Design review of the part built by this model. Coordinates are the model's own, in mm. Coordinates: 2 decimals unless noted, no trailing zeros. Write each loop counter-clockwise with the first axis right and the second up, starting at its lowest first coordinate (ties: lowest second). Pieces come first, ordered by that corner, then holes.
Q1. Add section A-A, the plane x = 0. Give the boundary of the cut face in (y, z).
Q2. To check wall thickness, follow probe 1 along Y at (x, z) = (0, 70); probe 2 along Z at (x, y) = (0, 1.25); probe 3 along Z at (x, y) = (1.5, 4). State the ranges of each line that lie inside material, in increasing order.
Q3. Add section B-B, the plane y = 5.25. Give the boundary of the cut face in (x, z).
Q4. Add section D-D, the plane z = 57. Give the boundary of the cut face in (x, y).
Q5. Clearance check with flat-ended pins moving along their axes: pin 1 Ø1.5 at (y, z) = (4, 46) entering from +X; pin 2 Ø1.5 at (y, z) = (-3, 41.5) entering from +X; pin 3 Ø2 at (x, z) = (0.5, 5) entering from +Y. State where each tip first meets the part, or that it passes through.
Q6. Add section C-C, the plane y = -0.75. Give the boundary of the cut face in (x, z), plus the area to 3 significant figures.
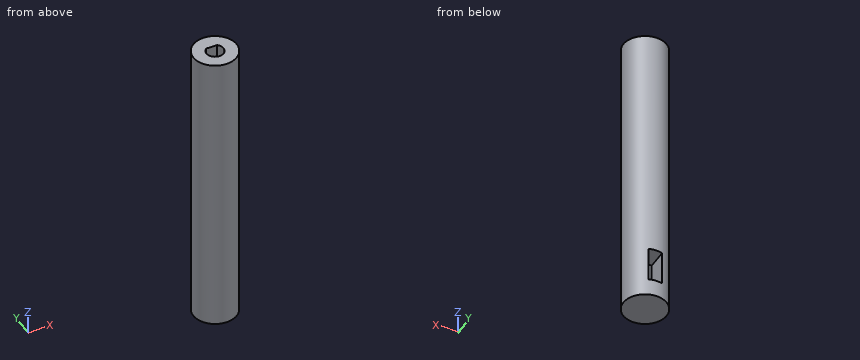
from build123d import *

# Parameters (mm, degrees)
BOSS_EXTRUDE1_DEPTH      = 80
BOSS_EXTRUDE1_DEPTH_BACK = 5
SKETCH1_R                = 6.3
CUT_EXTRUDE1_DEPTH       = 10
CUT_EXTRUDE3_DEPTH       = 17


with BuildPart() as part:
    # Sketch1 → Boss-Extrude1 (new, two sides: drawn at the far end of the back side and taken through both)
    with BuildSketch(Plane.XY.offset(-BOSS_EXTRUDE1_DEPTH_BACK)):
        Circle(SKETCH1_R)
    extrude(amount=BOSS_EXTRUDE1_DEPTH + BOSS_EXTRUDE1_DEPTH_BACK)

    # Sketch6 → Cut-Extrude1 (cut)
    with BuildSketch(Plane(origin=(0, 0, 0), x_dir=(1, 0, 0), z_dir=(0, 1, 0))):
        Polygon((0, 0), (-1.955160092, 0), (-1.955160092, -10), (2.038358394, -10), (2.038358394, 0), align=None)
    extrude(amount=CUT_EXTRUDE1_DEPTH, mode=Mode.SUBTRACT)

    # Sketch7 → Cut-Extrude3 (cut)
    with BuildSketch(Plane.XY.offset(80)):
        with BuildLine():
            Line((1.60670282, 1.915334448), (0, 1.915334448))
            Line((0, 1.915334448), (-1.60670282, 1.915334448))
            ThreePointArc((-1.60670282, 1.915334448), (-1.056703116, -2.265696035), (2.5, 0))
            ThreePointArc((2.5, 0), (2.265696035, 1.056703116), (1.60670282, 1.915334448))
        make_face()
    extrude(amount=-CUT_EXTRUDE3_DEPTH, mode=Mode.SUBTRACT)


solid = part.part
Here are the results:
1. outline: (-6.3, -5) - (6.3, -5) - (6.3, 0) - (0, 0) - (0, 10) - (6.3, 10) - (6.3, 80) - (1.92, 80) - (1.92, 63) - (-2.5, 63) - (-2.5, 80) - (-6.3, 80) - close
2. probe 1: y = -6.3 to -2.5, 1.92 to 6.3
2. probe 2: z = -5 to 0, 10 to 63
2. probe 3: z = -5 to 0, 10 to 80
3. outline: (-3.48, -5) - (3.48, -5) - (3.48, 80) - (-3.48, 80) - close; hole (-1.96, 0) - (2.04, 0) - (2.04, 10) - (-1.96, 10) - close
4. outline: circle Ø12.6 at (0, 0)
5. pin 1: stops at x = 5.4
5. pin 2: stops at x = 5.88
5. pin 3: stops at y = 0
6. outline: (-6.26, -5) - (6.26, -5) - (6.26, 80) - (2.38, 80) - (2.38, 63) - (-2.38, 63) - (-2.38, 80) - (-6.26, 80) - close
6. area: 982 mm2
